Work out the finished part from the listing and answer in its coordinate system (mm). Face numbers are marked on the shaded views. A direction names the side the tool comes from. Coordinates: 2 decimals unless noted, no trailing zeros. Order: outer loops, then holes, each group sorted by start corner. A loop starts at its lowest first (then second) coordinate and runs counter-clockwise, first axis right, second up. Notation, with made-up numbers: M 21.5,67 L 48.5,67 A15 ccw 48.5,75 Z; hole C 6,17.5 d9. An arc over 180 degrees is marked long. Use a Markdown table: item, result.
from build123d import *

# Parameters (mm, degrees)
EXTRUDE_1_DEPTH     = 6
SKETCH_2_R          = 1.5
CUT_EXTRUDE_1_DEPTH = 20.23763281
SKETCH_3_R          = 1.6
EXTRUDE_2_DEPTH     = 6
FILLET_1_R          = 2.1
FILLET_2_R          = 1
SKETCH_4_R          = 1.25
CUT_EXTRUDE_2_DEPTH = 20.979768962


with BuildPart() as part:
    # ｽｹｯﾁ1 → ﾎﾞｽ - 押し出し1 (new body)
    with BuildSketch(Plane.XY):
        with BuildLine():
            Line((-1.255, 5.918401389), (-1.255, 14.36257258))
            Line((-1.255, 14.36257258), (-3.255, 14.36257258))
            Line((-3.255, 14.36257258), (-3.255, 7.36257258))
            ThreePointArc((-3.255, 7.36257258), (0, -8.05), (3.255, 7.36257258))
            Line((3.255, 7.36257258), (3.255, 14.36257258))
            Line((3.255, 14.36257258), (1.255, 14.36257258))
            Line((1.255, 14.36257258), (1.255, 5.918401389))
            ThreePointArc((1.255, 5.918401389), (0, -6.05), (-1.255, 5.918401389))
        make_face()
    extrude(amount=EXTRUDE_1_DEPTH)

    # ｽｹｯﾁ2 → ｶｯﾄ - 押し出し1 (cut, through all)
    with BuildSketch(Plane(origin=(3.255, 0, 0), x_dir=(0, 0, -1), z_dir=(1, 0, 0))):
        with Locations(Location((-3, 11.56257258, 0), (0, 0, 90))):
            Circle(SKETCH_2_R)
    extrude(amount=-CUT_EXTRUDE_1_DEPTH, mode=Mode.SUBTRACT)

    # ｽｹｯﾁ3 → ﾎﾞｽ - 押し出し2 (add, through all)
    # profile 1 of 3: a face of its own
    with BuildSketch(Plane.XY.offset(6)):
        with BuildLine():
            Line((-4.969302513, 6.333129758), (-8.026279442, 8.098076211))
            ThreePointArc((-8.026279442, 8.098076211), (-12.124355653, 7), (-11.026279442, 2.901923789))
            Line((-11.026279442, 2.901923789), (-7.969302513, 1.136977336))
            ThreePointArc((-7.969302513, 1.136977336), (-6.9715045, 4.025), (-4.969302513, 6.333129758))
        make_face()
        with Locations((-9.526279442, 5.5)):
            Circle(SKETCH_3_R, mode=Mode.SUBTRACT)
    # profile 2 of 3: a face of its own
    with BuildSketch(Plane.XY.offset(6)):
        with BuildLine():
            Line((8.026279442, 8.098076211), (4.969302513, 6.333129758))
            ThreePointArc((4.969302513, 6.333129758), (6.9715045, 4.025), (7.969302513, 1.136977336))
            Line((7.969302513, 1.136977336), (11.026279442, 2.901923789))
            ThreePointArc((11.026279442, 2.901923789), (12.124355653, 7), (8.026279442, 8.098076211))
        make_face()
        with Locations((9.526279442, 5.5)):
            Circle(SKETCH_3_R, mode=Mode.SUBTRACT)
    # profile 3 of 3: a face of its own
    with BuildSketch(Plane.XY.offset(6)):
        with BuildLine():
            Line((3, -11), (3, -7.470107094))
            ThreePointArc((3, -7.470107094), (0, -8.05), (-3, -7.470107094))
            Line((-3, -7.470107094), (-3, -11))
            ThreePointArc((-3, -11), (0, -14), (3, -11))
        make_face()
        with Locations((0, -11)):
            Circle(SKETCH_3_R, mode=Mode.SUBTRACT)
    extrude(amount=-EXTRUDE_2_DEPTH)

    # ﾌｨﾚｯﾄ1
    # the kernel refuses this fillet: 2.1 mm, written as the material it adds along each edge
    with BuildSketch(Plane(origin=(3.255, 7.36257258, 0), x_dir=(0.8842030952275957, -0.46710265080594376, 0), z_dir=(0, 0, 1))) as fillet_1_piece_1:
        with BuildLine():
            CenterArc((1.268338995, 2.094894415), FILLET_1_R, 207.846387093, 58.157490839)
            Line((-0.588487505, 1.113978849), (0, 0))
            ThreePointArc((0, 0), (0.560996094, 0.019571407), (1.121992188, 0))
        make_face()
    extrude(amount=6)
    with BuildSketch(Plane(origin=(-3.255, 7.36257258, 0), x_dir=(0, 1, 0), z_dir=(0, 0, 1))) as fillet_1_piece_2:
        with BuildLine():
            CenterArc((1.25986762, 2.1), FILLET_1_R, 211.842509161, 58.157490839)
            ThreePointArc((-0.524085525, 0.992068966), (-0.244737664, 0.505176339), (0, 0))
            Line((0, 0), (1.25986762, 0))
        make_face()
    extrude(amount=6)
    with BuildSketch(Plane(origin=(-4.969302513, 6.333129758, 6), x_dir=(0.8292498658950391, 0.5588780367066322, 0), z_dir=(0, 0, -1)), Plane(origin=(7.969302513, 1.136977336, 6), x_dir=(0.06937764445759169, -0.9975904683032591, 0), z_dir=(0, 0, -1)), Plane(origin=(-3, -7.470107094, 6), x_dir=(-0.8986275103526323, 0.4387124315966321, 0), z_dir=(0, 0, -1))) as fillet_1_piece_3:
        with BuildLine():
            CenterArc((1.314348194, -2.094516792), FILLET_1_R, 94.141330549, 59.836911418)
            Line((-0.572769578, -1.173220685), (0, 0))
            ThreePointArc((0, 0), (0.581346317, -0.021018965), (1.162692633, 0))
        make_face()
    extrude(amount=6)
    with BuildSketch(Plane(origin=(-7.969302513, 1.136977336, 6), x_dir=(-0.06937764445760207, -0.9975904683032585, 0), z_dir=(0, 0, -1)), Plane(origin=(4.969302513, 6.333129758, 6), x_dir=(-0.8292498658950355, 0.5588780367066375, 0), z_dir=(0, 0, -1)), Plane(origin=(3, -7.470107094, 6), x_dir=(0.8986275103526384, 0.43871243159661977, 0), z_dir=(0, 0, -1))) as fillet_1_piece_4:
        with BuildLine():
            CenterArc((1.314348194, 2.094516792), FILLET_1_R, 206.021758033, 59.836911418)
            Line((-0.572769578, 1.173220685), (0, 0))
            ThreePointArc((0, 0), (0.581346317, 0.021018965), (1.162692633, 0))
        make_face()
    extrude(amount=6)

    # ﾌｨﾚｯﾄ2
    fillet_2_edges = [part.edges().sort_by_distance(p)[0] for p in [
        (1.255, 5.918401389, 3),
        (-1.255, 5.918401389, 3),
    ]]
    fillet(fillet_2_edges, radius=FILLET_2_R)

    # ｽｹｯﾁ4 → ｶｯﾄ - 押し出し2 (cut, through all)
    with BuildSketch(Plane.XY.offset(6)):
        with Locations((4.255, 11.49250639)):
            Circle(SKETCH_4_R)
        with Locations((-4.255, 11.49250639)):
            Circle(SKETCH_4_R)
    extrude(amount=-CUT_EXTRUDE_2_DEPTH, mode=Mode.SUBTRACT)


solid = part.part
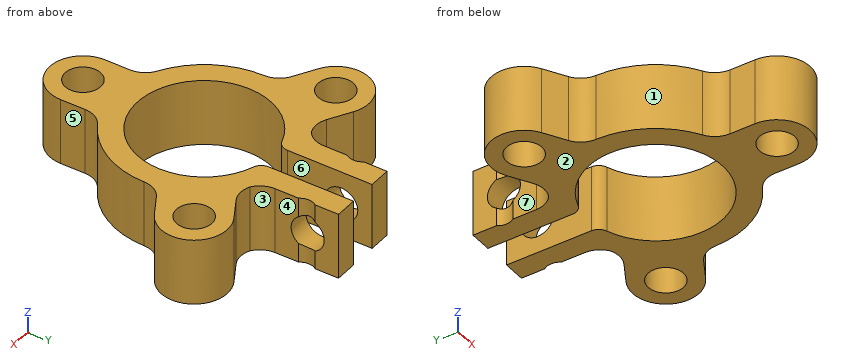
(1) Given P1, Ø2.5, axis at y = 13.5, z = 3.5, coming from the +X side (3 decimals); P2, Ø2.5, axis at y = -9.5, z = 3.5, coming from the +X side; P3, Ø2.5, axis at y = 9.5, z = 4.5, coming from the -X side, each flat-ended and moving along its own axis, determine where each tip first touches the part or whether it passes through.
Conclusion:
| item | result |
|---|---|
| P1 | x = 3.255 |
| P2 | x = 3.07 |
| P3 | x = -10.73 |
(2) Which of the six approach directions +Z, -Z, +X, -X, +Y, -Y give full straight-line access (tool end or side, diameter ignored) to the marked faces 5, 6 and 7?
Conclusion:
| item | result |
|---|---|
| face 5 | +Z, -Z, +X, -Y |
| face 6 | +Z, -Z, +Y |
| face 7 | +Z, -Z, -X, +Y |
(3) A cutting plane is placed at B-B (y = -4.25). Determine the outline of the cut face in (x, z).
Conclusion:
| item | result |
|---|---|
| outline | M -6.84,0 L -4.31,0 L -4.31,6 L -6.84,6 Z; M 4.31,0 L 6.84,0 L 6.84,6 L 4.31,6 Z |
(4) A cutting plane is placed at A-A (x = -2.25). Determine the outline of the cut face in (y, z).
Conclusion:
| item | result |
|---|---|
| outline | M -12.98,0 L -5.62,0 L -5.62,6 L -12.98,6 Z; M 5.62,0 L 14.36,0 L 14.36,6 L 5.62,6 Z; hole C 11.56,3 d3 |
(5) Determine the mould class of the marked faces 1, 2, 3 and 4 for opening direction X: pulls with the +X half, pulls with the -X half, needs draft (parallel to the pull), parting line crosses it, or undercut.
Conclusion:
| item | result |
|---|---|
| face 1 | pulls with the -X half |
| face 2 | needs draft |
| face 3 | undercut |
| face 4 | pulls with the +X half |
(6) A cutting plane is placed at C-C (z = 3). Give the number of separate pieces and of enclosed holes in the cut face, then the cut area to 3 significant figures.
Conclusion:
| item | result |
|---|---|
| separate pieces | 3 |
| enclosed holes | 3 |
| area | 175 mm2 |
(7) Straight lines are drawn through the part: L1, parallel to X at y = 9, z = 5.5 (3 decimals); L2, parallel to X at y = 0, z = 3.85; L3, parallel to X at y = 7.5, z = 1 (3 decimals). For each, find the intervals that lie inside material, in ascending order.
Conclusion:
| item | result |
|---|---|
| L1 | -3.255 to -1.255, 1.255 to 3.255 |
| L2 | -8.05 to -6.05, 6.05 to 8.05 |
| L3 | -11.762 to -6.99, -3.58 to -1.255, 1.255 to 3.58, 6.99 to 11.762 |
